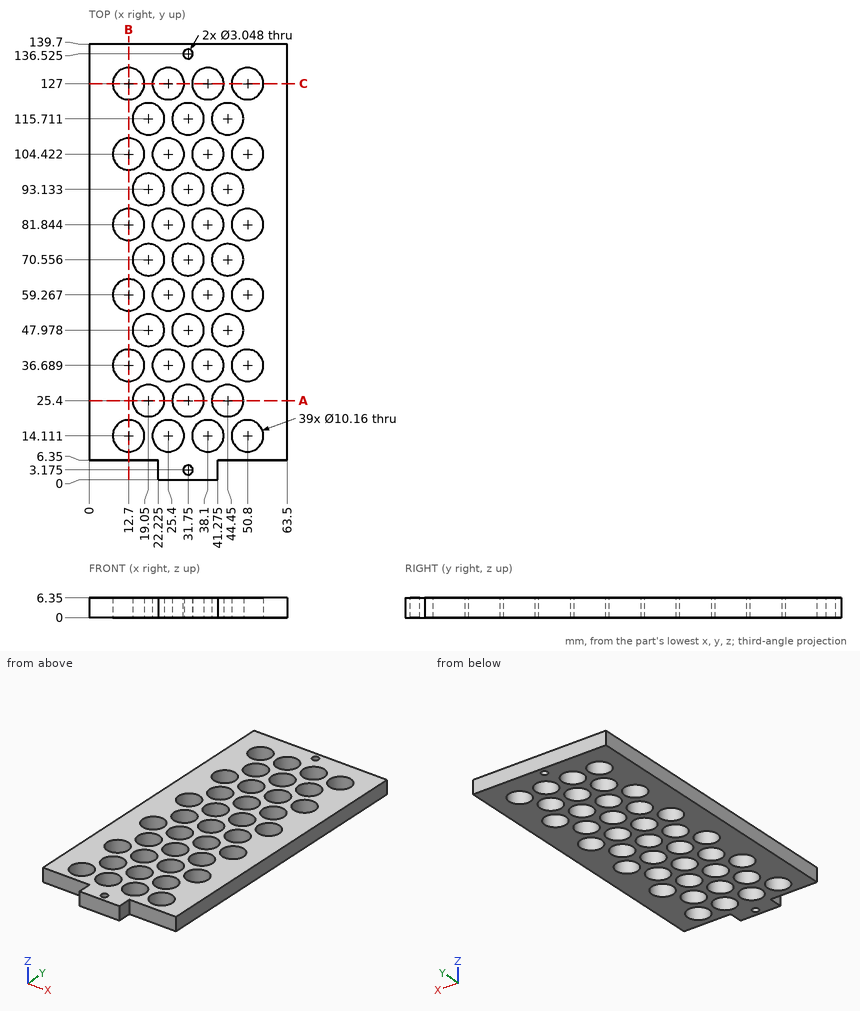
Geometry: see drawing. Coordinates: mm, zero at the bounding-box minimum. Round coordinates to 2 decimals unless told otherwise and drop trailing zeros. Loops run counter-clockwise (first coordinate to the right, second up) from the corner with the lowest first, then second, coordinate; pieces in that order, holes last. Notation, with made-up numbers: M 14,81 L 29,81 A27 ccw 29,119 Z; hole C -7.5,34.5 d1. An arc over 180 degrees is marked long. Use a Markdown table: item, result. Add a question column.
1. Ray query, line 1 along X through (y, z) = (93, 3); line 2 along X through (y, z) = (32.5, 0.5) (1 decimal); line 3 along X through (y, z) = (129, 4.75). Return the intervals inside material, ascending. Write a range as [from, to].
2. Cut plane A-A, the plane y = 25.4. Output: boundary loops of the cut face in (x, z).
3. Cut plane C-C, the plane y = 127. Output: boundary loops of the cut face in (x, z).
4. Contact query for flat-ended pins moving along their axis: pin 1 (8 mm diameter, centred on x = 12.7, y = 104.42, fed in from +Z); pin 2 (3 mm diameter, centred on x = 49.5, z = 2.5, fed in from -Y). Output: stop coordinate, or through.
5. Cut plane B-B, the plane x = 12.7. State how many separate pieces and enclosed holes the cut face has.
Solution:
| question | item | result |
|---|---|---|
| 1 | line 1 | x = [0, 13.97], [24.13, 26.67], [36.83, 39.37], [49.53, 63.5] |
| 1 | line 2 | x = [0, 9.8], [15.6, 22.5], [28.3, 35.2], [41, 47.9], [53.7, 63.5] |
| 1 | line 3 | x = [0, 8.03], [17.37, 20.73], [30.07, 33.43], [42.77, 46.13], [55.47, 63.5] |
| 2 | outline | M 0,0 L 13.97,0 L 13.97,6.35 L 0,6.35 Z; M 24.13,0 L 26.67,0 L 26.67,6.35 L 24.13,6.35 Z; M 36.83,0 L 39.37,0 L 39.37,6.35 L 36.83,6.35 Z; M 49.53,0 L 63.5,0 L 63.5,6.35 L 49.53,6.35 Z |
| 3 | outline | M 0,0 L 7.62,0 L 7.62,6.35 L 0,6.35 Z; M 17.78,0 L 20.32,0 L 20.32,6.35 L 17.78,6.35 Z; M 30.48,0 L 33.02,0 L 33.02,6.35 L 30.48,6.35 Z; M 43.18,0 L 45.72,0 L 45.72,6.35 L 43.18,6.35 Z; M 55.88,0 L 63.5,0 L 63.5,6.35 L 55.88,6.35 Z |
| 4 | pin 1 | passes through |
| 4 | pin 2 | stops at y = 6.35 |
| 5 | separate pieces | 7 |
| 5 | enclosed holes | 0 |
